Source: CAD feature listing. Evaluate the final solid. Frame: model axes, mm. Coordinates: 2 decimals unless noted, no trailing zeros. Loops run counter-clockwise (first coordinate to the right, second up) from the corner with the lowest first, then second, coordinate; pieces in that order, holes last. Notation, with made-up numbers: (-24, -16) -> (32, -16) arc R24 ccw to (32, 14) -> close; hole circle Ø11 at (-7, 12). An arc over 180 degrees is marked (long way). One line per question, with ' | ' between items. Start each with the question number.
```python
from build123d import *

# Parameters (mm, degrees)
BOSS_EXTRUDE1_DEPTH = 2.5
SKETCH2_R           = 1.5
CUT_EXTRUDE1_DEPTH  = 142.178079035
SKETCH3_R           = 1.6
CUT_EXTRUDE2_DEPTH  = 10
SKETCH4_R           = 1.6
CUT_EXTRUDE3_DEPTH  = 10
SKETCH5_R           = 1.6
CUT_EXTRUDE4_DEPTH  = 10
SKETCH8_R           = 1.6
CUT_EXTRUDE5_DEPTH  = 10
SKETCH9_R           = 1.7
CUT_EXTRUDE6_DEPTH  = 10
SKETCH10_R          = 7.5
CUT_EXTRUDE7_DEPTH  = 10


with BuildPart() as part:
    # Sketch1 → Boss-Extrude1 (new body)
    with BuildSketch(Plane(origin=(0, 0, 0), x_dir=(1, 0, 0), z_dir=(0, 1, 0))):
        with BuildLine():
            Line((10, 0), (120, 0))
            ThreePointArc((120, 0), (127.071067812, 2.928932188), (130, 10))
            Line((130, 10), (130, 45))
            ThreePointArc((130, 45), (127.071067812, 52.071067812), (120, 55))
            Line((120, 55), (10, 55))
            ThreePointArc((10, 55), (2.928932188, 52.071067812), (0, 45))
            Line((0, 45), (0, 10))
            ThreePointArc((0, 10), (2.928932188, 2.928932188), (10, 0))
        make_face()
    extrude(amount=BOSS_EXTRUDE1_DEPTH)

    # Sketch2 → Cut-Extrude1 (cut, through all)
    with BuildSketch(Plane(origin=(0, 2.5, 0), x_dir=(1, 0, 0), z_dir=(0, 1, 0))):
        with Locations(Location((14, 5, 0), (0, 0, 270))):
            Circle(SKETCH2_R)
        with Locations(Location((14, 50, 0), (0, 0, 270))):
            Circle(SKETCH2_R)
        with Locations(Location((116, 5, 0), (0, 0, 90))):
            Circle(SKETCH2_R)
        with Locations(Location((116, 50, 0), (0, 0, 90))):
            Circle(SKETCH2_R)
    extrude(amount=-CUT_EXTRUDE1_DEPTH, mode=Mode.SUBTRACT)

    # Sketch3 → Cut-Extrude2 (cut)
    with BuildSketch(Plane(origin=(0, 2.5, 0), x_dir=(1, 0, 0), z_dir=(0, 1, 0))):
        with Locations(Location((12, 33, 0), (0, 0, 270))):
            Circle(SKETCH3_R)
    extrude(amount=-CUT_EXTRUDE2_DEPTH, mode=Mode.SUBTRACT)

    # Sketch4 → Cut-Extrude3 (cut)
    with BuildSketch(Plane(origin=(0, 2.5, 0), x_dir=(1, 0, 0), z_dir=(0, 1, 0))):
        with Locations(Location((12, 22, 0), (0, 0, 270))):
            Circle(SKETCH4_R)
    extrude(amount=-CUT_EXTRUDE3_DEPTH, mode=Mode.SUBTRACT)

    # Sketch5 → Cut-Extrude4 (cut)
    with BuildSketch(Plane(origin=(0, 2.5, 0), x_dir=(1, 0, 0), z_dir=(0, 1, 0))):
        with Locations(Location((32, 33, 0), (0, 0, 270))):
            Circle(SKETCH5_R)
        with Locations(Location((32, 22, 0), (0, 0, 270))):
            Circle(SKETCH5_R)
    extrude(amount=-CUT_EXTRUDE4_DEPTH, mode=Mode.SUBTRACT)

    # Sketch8 → Cut-Extrude5 (cut)
    with BuildSketch(Plane(origin=(0, 2.5, 0), x_dir=(1, 0, 0), z_dir=(0, 1, 0))):
        with Locations(Location((98, 33, 0), (0, 0, 270))):
            Circle(SKETCH8_R)
        with Locations(Location((98, 22, 0), (0, 0, 270))):
            Circle(SKETCH8_R)
        with Locations(Location((118, 33, 0), (0, 0, 270))):
            Circle(SKETCH8_R)
        with Locations(Location((118, 22, 0), (0, 0, 270))):
            Circle(SKETCH8_R)
    extrude(amount=-CUT_EXTRUDE5_DEPTH, mode=Mode.SUBTRACT)

    # Sketch9 → Cut-Extrude6 (cut)
    with BuildSketch(Plane(origin=(0, 2.5, 0), x_dir=(1, 0, 0), z_dir=(0, 1, 0))):
        with Locations(Location((32.5, 50, 0), (0, 0, 270))):
            Circle(SKETCH9_R)
        with Locations(Location((97.5, 50, 0), (0, 0, 270))):
            Circle(SKETCH9_R)
        with Locations(Location((97.5, 5, 0), (0, 0, 270))):
            Circle(SKETCH9_R)
        with Locations(Location((32.5, 5, 0), (0, 0, 270))):
            Circle(SKETCH9_R)
    extrude(amount=-CUT_EXTRUDE6_DEPTH, mode=Mode.SUBTRACT)

    # Sketch10 → Cut-Extrude7 (cut)
    with BuildSketch(Plane.XZ):
        with Locations(Location((22, -27.5, 0), (0, 0, 270))):
            Circle(SKETCH10_R)
        with Locations(Location((108, -27.5, 0), (0, 0, 90))):
            Circle(SKETCH10_R)
    extrude(amount=-CUT_EXTRUDE7_DEPTH, mode=Mode.SUBTRACT)


solid = part.part
```
(1) Cut plane B-B, the plane y = 1.9. State how many separate pieces and enclosed holes the cut face has, and give its area (3 significant figures).
(2) Draft query along Z for faces 1 (the flat face through (64, 1, 0)), 2 (the cylindrical face through (14.07, 1.27, -6.5)), 3 (the cylindrical face through (98.07, 1.27, -34.6)), 4 (the cylindrical face through (3.01, 1.23, -52.15)). Return one class per face: pulls with the +Z half, pulls with the -Z half, needs draft (parallel to the pull), parting line crosses it, or undercut.
(3) Ray query, L1, parallel to X at y = 1.6, z = -27.5; L2, parallel to Z at x = 118, y = 2.25; L3, parallel to Z at x = 116, y = 1.25. Return the intervals inside material, ascending.
(4) Cut plane C-C, the plane x = 104.5. Return the cut outline in (y, z), and give its area (3 significant figures).
(5) Cut plane A-A, the plane z = -22. Return the cut outline in (x, y), and give its area (3 significant figures).
(6) Contact query for a flat-ended pin moving along its axis: pin 1 Ø2.5 at (x, z) = (116, -50) entering from +Y (3 decimals). Output: stop coordinate, or through.
Here are the results:
1) separate pieces: 1 | enclosed holes: 18 | area: 6,580 mm2
2) face 1: pulls with the +Z half | face 2: undercut | face 3: undercut | face 4: pulls with the -Z half
3) L1: x = 0 to 14.5, 29.5 to 100.5, 115.5 to 130 | L2: z = -55 to -34.6, -31.4 to -23.6, -20.4 to 0 | L3: z = -55 to -51.5, -48.5 to -6.5, -3.5 to 0
4) outline: (0, -55) -> (2.5, -55) -> (2.5, -34.13) -> (0, -34.13) -> close; (0, -20.87) -> (2.5, -20.87) -> (2.5, 0) -> (0, 0) -> close | area: 104 mm2
5) outline: (0, 0) -> (10.4, 0) -> (10.4, 2.5) -> (0, 2.5) -> close; (13.6, 0) -> (16.9, 0) -> (16.9, 2.5) -> (13.6, 2.5) -> close; (27.1, 0) -> (30.4, 0) -> (30.4, 2.5) -> (27.1, 2.5) -> close; (33.6, 0) -> (96.4, 0) -> (96.4, 2.5) -> (33.6, 2.5) -> close; (99.6, 0) -> (102.9, 0) -> (102.9, 2.5) -> (99.6, 2.5) -> close; (113.1, 0) -> (116.4, 0) -> (116.4, 2.5) -> (113.1, 2.5) -> close; (119.6, 0) -> (130, 0) -> (130, 2.5) -> (119.6, 2.5) -> close | area: 242 mm2
6) pin 1: passes through
